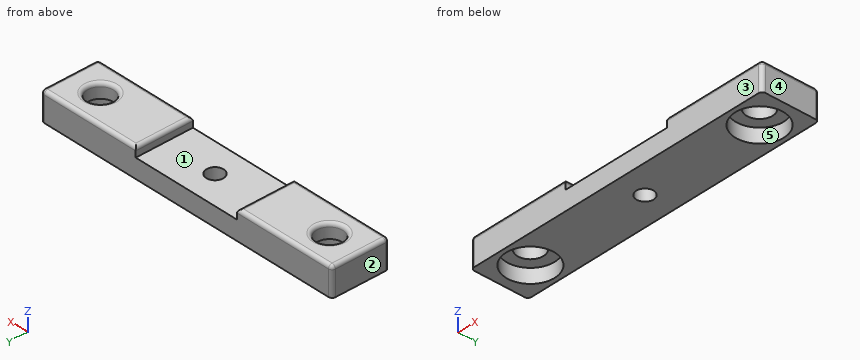
```python
from build123d import *

# Parameters (mm, degrees)
ESQUISSE2_W             = 66
ESQUISSE2_H             = 12
BOSS_EXTRU_1_DEPTH      = 6
ESQUISSE3_W             = 23
ESQUISSE3_H             = 12
ENL_V_MAT_EXTRU_1_DEPTH = 2
ESQUISSE4_R             = 1.8
ENL_V_MAT_EXTRU_2_DEPTH = 5
ESQUISSE5_R             = 2.75
ENL_V_MAT_EXTRU_3_DEPTH = 7
ESQUISSE6_R             = 5.1
ENL_V_MAT_EXTRU_4_DEPTH = 3
CONG_1_R                = 0.75


with BuildPart() as part:
    # Esquisse2 → Boss.-Extru.1 (new body)
    with BuildSketch(Plane.XY):
        with Locations((33, 6)):
            Rectangle(ESQUISSE2_W, ESQUISSE2_H)
    extrude(amount=BOSS_EXTRU_1_DEPTH)

    # Esquisse3 → Enlèv. mat.-Extru.1 (cut)
    with BuildSketch(Plane.XY.offset(6)):
        with Locations((33, 6)):
            Rectangle(ESQUISSE3_W, ESQUISSE3_H)
    extrude(amount=-ENL_V_MAT_EXTRU_1_DEPTH, mode=Mode.SUBTRACT)

    # Esquisse4 → Enlèv. mat.-Extru.2 (cut, through all)
    with BuildSketch(Plane.XY.offset(4)):
        with Locations((33, 6)):
            Circle(ESQUISSE4_R)
    extrude(amount=-ENL_V_MAT_EXTRU_2_DEPTH, mode=Mode.SUBTRACT)

    # Esquisse5 → Enlèv. mat.-Extru.3 (cut, through all)
    with BuildSketch(Plane(origin=(0, 0, 0), x_dir=(-1, 0, 0), z_dir=(0, 0, -1))):
        with Locations((-59, 6)):
            Circle(ESQUISSE5_R)
        with Locations((-7, 6)):
            Circle(ESQUISSE5_R)
    extrude(amount=-ENL_V_MAT_EXTRU_3_DEPTH, mode=Mode.SUBTRACT)

    # Esquisse6 → Enlèv. mat.-Extru.4 (cut)
    with BuildSketch(Plane(origin=(0, 0, 0), x_dir=(-1, 0, 0), z_dir=(0, 0, -1))):
        with Locations((-59, 6)):
            Circle(ESQUISSE6_R)
        with Locations((-7, 6)):
            Circle(ESQUISSE6_R)
    extrude(amount=-ENL_V_MAT_EXTRU_4_DEPTH, mode=Mode.SUBTRACT)

    # Congé1
    cong_1_edges = [part.edges().sort_by_distance(p)[0] for p in [
        (66, 6, 6),
        (55.25, 12, 6),
        (55.25, 0, 6),
        (10.75, 12, 6),
        (21.5, 6, 6),
        (44.5, 6, 6),
        (61.75, 6, 6),
        (0, 6, 6),
        (9.75, 6, 6),
        (10.75, 0, 6),
        (0, 12, 3),
        (66, 12, 3),
        (66, 0, 3),
        (0, 0, 3),
    ]]
    fillet(cong_1_edges, radius=CONG_1_R)


solid = part.part
```
Build history of the part. All positions in model axes, mm. Face numbers are marked on the shaded views. A direction names the side the tool comes from. Round coordinates to 2 decimals unless told otherwise and drop trailing zeros. Loops run counter-clockwise (first coordinate to the right, second up) from the corner with the lowest first, then second, coordinate; pieces in that order, holes last.
Item 1: Saw through at C-C (x = 33). List the corners of the cut face in (y, z), then the cut area to 3 significant figures.
Item 2: Drill centre lines: line 1 along X through (y, z) = (7.5, 5.25); line 2 along X through (y, z) = (10.5, 1.1); line 3 along Y through (x, z) = (59, 2). Where is each one in solid material? Low to high.
Item 3: Which spindle directions (+Z, -Z, +X, -X, +Y, -Y) get a long thin tool onto all of the face, cutting with end or side? Do the marked faces 4 and 5. Say none if no direction does.
Item 4: Pin check, flat tips, straight feed: P1, Ø6.5, axis at x = 7, y = 6, coming from the +Z side; P2, Ø3, axis at x = 5.5, y = 8.5, coming from the -Z side. Stop position of each tip, or through.
Item 5: Saw through at D-D (y = 6). State how many separate pieces and enclosed holes the cut face has, then the cut area to 3 significant figures.
Item 6: Two-plate mould, pull along X, no slides. Class the marked faces 1, 2 and 3: released by +X, released by -X, zero draft, split by the parting line, or undercut.
Item 7: Saw through at A-A (x = 7). List the corners of the cut face in (y, z), then the cut area to 3 significant figures.
Item 8: Saw through at B-B (z = 1.85). List the corners of the cut face in (x, y), then the cut area to 3 significant figures.
Worked answers:
1. outline: (0, 0) - (4.2, 0) - (4.2, 4) - (0, 4) - close; (7.8, 0) - (12, 0) - (12, 4) - (7.8, 4) - close
1. area: 33.6 mm2
2. line 1: x = 0 to 4.7, 9.3 to 21.5, 44.5 to 56.7, 61.3 to 66
2. line 2: x = 0 to 4.6, 9.4 to 56.6, 61.4 to 66
2. line 3: y = 0 to 0.9, 11.1 to 12
3. face 4: +Z, -Z, +X, +Y, -Y
3. face 5: -Z
4. P1: stops at z = 5.96
4. P2: stops at z = 3
5. separate pieces: 4
5. enclosed holes: 0
5. area: 240 mm2
6. face 1: undercut
6. face 2: released by -X
6. face 3: zero draft
7. outline: (0, 0) - (0.9, 0) - (0.9, 3) - (3.25, 3) - (3.25, 5.25) arc R0.75 ccw to (2.5, 6) - (0.75, 6) arc R0.75 ccw to (0, 5.25) - close; (8.75, 3) - (11.1, 3) - (11.1, 0) - (12, 0) - (12, 5.25) arc R0.75 ccw to (11.25, 6) - (9.5, 6) arc R0.75 ccw to (8.75, 5.25) - close
7. area: 24.4 mm2
8. outline: (0, 0.75) arc R0.75 ccw to (0.75, 0) - (65.25, 0) arc R0.75 ccw to (66, 0.75) - (66, 11.25) arc R0.75 ccw to (65.25, 12) - (0.75, 12) arc R0.75 ccw to (0, 11.25) - close; hole circle Ø10.2 at (7, 6); hole circle Ø3.6 at (33, 6); hole circle Ø10.2 at (59, 6)
8. area: 618 mm2
